Autodesk Inventor part; units mm, degrees
ref_plane "YZ Plane" through (0, 0, 0) normal (1, 0, 0) x (0, 1, 0)
ref_plane "XZ Plane" through (0, 0, 0) normal (0, 1, 0) x (-1, 0, 0)
ref_plane "XY Plane" through (0, 0, 0) normal (0, 0, 1) x (1, 0, 0)
sketch "Sketch1" plane through (0, 0, 0) normal (0, 0, 1) x (1, 0, 0)
  line L0 (0, 0) -> (0, 9.712)
  line L1 (0, 9.712) -> (14.5, 24.212)
  line L2 (14.5, 24.212) -> (149.675, 24.212)
  line L3 (0, 0) -> (149.675, 0)
  circle A0 centre (10.1, 8) radius 3
  line L4 (149.675, 42.0637) -> (149.675, 59.6175)
  line L5 (299.35, 0) -> (299.35, 9.712)
  line L6 (299.35, 9.712) -> (284.85, 24.212)
  line L7 (284.85, 24.212) -> (149.675, 24.212)
  line L8 (299.35, 0) -> (149.675, 0)
  circle A1 centre (289.25, 8) radius 3
  dimension "d0" = 135
  dimension "d1" = 149.675
  dimension "d2" = 9.712
  dimension "d3" = 24.212
  dimension "d4" = 6
  dimension "d5" = 8
  dimension "d6" = 10.1
extrude "Extrusion1" add sketch "Sketch1" along normal blind 5
properties part number "road"
Build history of the part. All positions in model axes, mm. Coordinates: 2 decimals unless noted, no trailing zeros. Order: outer loops, then holes, each group sorted by start corner. A loop starts at its lowest first (then second) coordinate and runs counter-clockwise, first axis right, second up. Notation, with made-up numbers: (24.25, 5) - (55.25, 5) arc R13 ccw to (55.25, 29) - close; hole circle Ø6 at (-25.75, 20.5). An arc over 180 degrees is marked (long way). Put each result on its own line as item: value.
1. Saw through at C-C (y = 18). Write the cut outline in (x, z).
Answer sheet:
outline: (8.29, 0) - (291.06, 0) - (291.06, 5) - (8.29, 5) - close
2. Saw through at B-B (x = 289.25). Write the cut outline in (y, z).
Answer sheet:
outline: (0, 0) - (5, 0) - (5, 5) - (0, 5) - close; (11, 0) - (19.81, 0) - (19.81, 5) - (11, 5) - close
3. Drop a flat-ended pin along its axis: P1, Ø3.5, axis at x = 10.1, y = 8, coming from the +Z side. Give the stop position or say it passes through.
Answer sheet:
P1: passes through
4. Probe line 1 along X through (y, z) = (8.75, 3.6); line 2 along Y through (x, z) = (289.25, 1.3); line 3 along Y through (x, z) = (12.5, 0.7). List the from-to ranges inside material, lowest first. Write a range as [from, to].
Answer sheet:
line 1: x = [0, 7.2], [13, 286.35], [292.15, 299.35]
line 2: y = [0, 5], [11, 19.81]
line 3: y = [0, 6.2], [9.8, 22.21]
5. Saw through at A-A (z = 3.7). Write the cut outline in (x, y).
Answer sheet:
outline: (0, 0) - (299.35, 0) - (299.35, 9.71) - (284.85, 24.21) - (14.5, 24.21) - (0, 9.71) - close; hole circle Ø6 at (10.1, 8); hole circle Ø6 at (289.25, 8)
6. Pull direction Y, two halves, no side cores. Call faces 1 (the face through (286.253, 7.868, 2.465)), 2 (the face through (7.89, 5.97, 2.46)), 3 (the face through (152, 0, 2)), 4 (the face through (292.2, 16.86, 2.46)): pulls with the +Y half, pulls with the -Y half, needs draft (parallel to the pull), parting line crosses it, or undercut.
Answer sheet:
face 1: undercut
face 2: undercut
face 3: pulls with the -Y half
face 4: pulls with the +Y half
